Geometry: final body of the model. Coordinates: model frame, mm. A direction names the side the tool comes from. Give positions to 0.01 mm unless a question says otherwise; leave off trailing zeros. Write each loop counter-clockwise with the first axis right and the second up, starting at its lowest first coordinate (ties: lowest second). Pieces come first, ordered by that corner, then holes. Notation, with made-up numbers: M -9.5,64 L 39.5,64 A11 ccw 39.5,79 Z; hole C 89,-23 d10. An arc over 180 degrees is marked long. Use one line per item in the form item = value. Start each with the question number.
Item 1: Access query for faces 1 (the flat face through (7, 19.15, 3)), 2 (the flat face through (16, 14, 6)), 3 (the flat face through (7, 11.15, 3)). Directions: +Z, -Z, +X, -X, +Y, -Y. A direction counts if a zero-diameter tool reaches every point of the face in a straight line with its end or side. Return the directions, or none.
Item 2: Pull-direction query (Y, two-part tool) for faces 4 (the cylindrical face through (21.001, 24.763, 0.76)), 5 (the flat face through (21.7, 0, 1)), 6 (the cylindrical face through (19.369, 0.526, 0.76)); classes: released by +Y, released by -Y, zero draft, split by the parting line, or undercut.
Item 3: Section query D-D on y = 13. Return loops of the section in (x, z), then the cut area to 3 significant figures.
Item 4: Contact query for flat-ended pins moving along their axis: P1, Ø1, axis at x = 3, y = 14, coming from the +Z side; P2, Ø1.2, axis at x = 6.5, z = 3, coming from the +Y side; P3, Ø12, axis at x = 8.5, y = -0.5, coming from the -Z side; P4, Ø1.2, axis at x = 7, z = 4.5, coming from the -Y side. Output: stop coordinate, or through.
Item 5: Section query B-B on x = -17.7. Return loops of the section in (y, z), then the cut area to 4 significant figures.
Item 6: Material intervals for line 1 along Y through (x, z) = (-17.7, 0.6); line 2 along Y through (x, z) = (17, 5.75); line 3 along Z through (x, y) = (2.5, 17), sorted ascending. Write a range as from..to.
Item 7: Section query A-A on y = 0. Return loops of the section in (x, z).
Item 8: Section query C-C on x = 13. Return loops of the section in (y, z), then the cut area to 3 significant figures.
from build123d import *

# Parameters (mm, degrees)
F0_W      = 43.4
F0_H      = 51
F1_DEPTH  = 1.5
F2_R      = 2.45
F3_R      = 1.75
F4_DEPTH  = 1.501
F5_W      = 9.5
F5_H      = 9.5
F6_DEPTH  = 4.5
F6_TAPER  = 1.5
F7_W      = 7.85
F7_H      = 4.95
F8_DEPTH  = 8.5
F9_W      = 4.25
F9_H      = 8
F10_DEPTH = 4.15
F12_DEPTH = 44.651
F13_DEPTH = 8.5


with BuildPart() as f1:
    # F0 (on Top) → F1 (new body)
    with BuildSketch(Plane.XY):
        Rectangle(F0_W, F0_H)
    extrude(amount=F1_DEPTH)

    # F2
    f2_edges = [f1.edges().sort_by_distance(p)[0] for p in [
        (-21.7, 25.5, 0.75),
        (21.7, 25.5, 0.75),
        (21.7, -25.5, 0.75),
        (-21.7, -25.5, 0.75),
    ]]
    fillet(f2_edges, radius=F2_R)

    # F3 (on face) → F4 (cut, through all)
    with BuildSketch(Plane.XY.offset(1.5)):
        with Locations((-17.7, 0)):
            Circle(F3_R)
        with Locations((17.7, 0)):
            Circle(F3_R)
    extrude(amount=-F4_DEPTH, mode=Mode.SUBTRACT)

    # F5 (on face) → F6 (join)
    with BuildSketch(Plane.XY.offset(1.5)):
        with Locations((15.95, 14.15)):
            Rectangle(F5_W, F5_H)
    extrude(amount=F6_DEPTH, taper=F6_TAPER)

    # F7 (on face) → F8 (join)
    with BuildSketch(Plane.XY.offset(1.5)):
        with Locations((-15.775, -20.075)):
            Rectangle(F7_W, F7_H)
    extrude(amount=F8_DEPTH)

    # F9 (on face) → F10 (join)
    with BuildSketch(Plane.XY.offset(1.5)):
        with Locations((6.725, 15.15)):
            Rectangle(F9_W, F9_H)
    extrude(amount=F10_DEPTH)

    # F11 (on face) → F12 (cut, through all)
    with BuildSketch(Plane(origin=(0, 19.15, 0), x_dir=(-1, 0, 0), z_dir=(0, 1, 0))):
        with BuildLine():
            ThreePointArc((-7.190682743, 1.55), (-7.9935060714, 5.0634608153), (-4.7462730221, 3.5))
            ThreePointArc((-4.7462730221, 3.5), (-5.1828122069, 2.2527669508), (-6.3018633013, 1.55))
            Line((-6.3018633013, 1.55), (-6.3018633013, 1.5))
            Line((-6.3018633013, 1.5), (-4.6, 1.5))
            Line((-4.6, 1.5), (-4.6, 5.65))
            Line((-4.6, 5.65), (-8.85, 5.65))
            Line((-8.85, 5.65), (-8.85, 1.5))
            Line((-8.85, 1.5), (-7.190682743, 1.5))
            Line((-7.190682743, 1.5), (-7.190682743, 1.55))
        make_face()
    extrude(amount=-F12_DEPTH, mode=Mode.SUBTRACT)

    # F13 (cut, through all): a face of the model
    f13_faces = [f1.faces().sort_by_distance(p)[0] for p in [
        (-15.775, -20.075, 10),
    ]]
    extrude(f13_faces, amount=-F13_DEPTH, mode=Mode.SUBTRACT)


solid = f1.part
Answer sheet:
q1.face_1 = +Z, +X, -X, +Y
q1.face_2 = +Z, +X, -X, +Y, -Y
q1.face_3 = +Z, -X, -Y
q2.face_4 = released by +Y
q2.face_5 = zero draft
q2.face_6 = undercut
q3.outline = M -21.7,0 L 21.7,0 L 21.7,1.5 L 20.7,1.5 L 20.58,6 L 11.32,6 L 11.2,1.5 L 7.19,1.5 L 7.19,1.55 A2 ccw long 6.3,1.55 L 6.3,1.5 L -21.7,1.5 Z
q3.area = 120 mm2
q4.P1 = 1.5
q4.P2 = 19.15
q4.P3 = 0
q4.P4 = 11.15
q5.outline = M -25.5,0 L -1.75,0 L -1.75,1.5 L -25.5,1.5 Z; M 1.75,0 L 25.5,0 L 25.5,1.5 L 1.75,1.5 Z
q5.area = 71.25 mm2
q6.line_1 = -25.5..-1.75, 1.75..25.5
q6.line_2 = 9.51..18.79
q6.line_3 = 0..1.5
q7.outline = M -21.7,0 L -19.45,0 L -19.45,1.5 L -21.7,1.5 Z; M -15.95,0 L 15.95,0 L 15.95,1.5 L -15.95,1.5 Z; M 19.45,0 L 21.7,0 L 21.7,1.5 L 19.45,1.5 Z
q8.outline = M -25.5,0 L 25.5,0 L 25.5,1.5 L 18.9,1.5 L 18.78,6 L 9.52,6 L 9.4,1.5 L -25.5,1.5 Z
q8.area = 119 mm2
